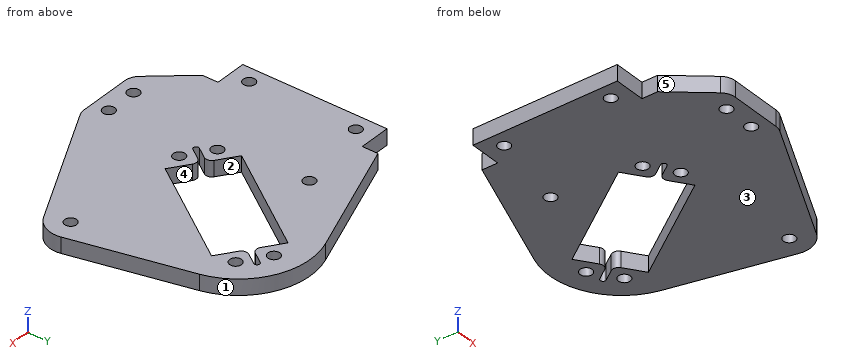
from build123d import *

# Parameters (mm, degrees)
ESQUISSE1_R        = 1.9
BOSS_EXTRU_1_DEPTH = 5


with BuildPart() as part:
    # Esquisse1 → Boss.-Extru.1 (new body)
    with BuildSketch(Plane.XY):
        with BuildLine():
            Line((40.548338426, -21.276277818), (-0.975727052, -42.264773686))
            ThreePointArc((-0.975727052, -42.264773686), (-2.030907408, -42.633295828), (-3.141586831, -42.758217285))
            Line((-3.141586831, -42.758217285), (-19.618188193, -42.758217285))
            ThreePointArc((-19.618188193, -42.758217285), (-21.685859542, -42.310660648), (-23.383370665, -41.048112535))
            Line((-23.383370665, -41.048112535), (-33.519906154, -28.967859949))
            Line((-33.519906154, -28.967859949), (-33.519906154, -23.969415955))
            Line((-33.519906154, -23.969415955), (-43.519906154, -23.969415955))
            Line((-43.519906154, -23.969415955), (-43.519906154, 22.030584045))
            Line((-43.519906154, 22.030584045), (-33.519906154, 22.030584045))
            Line((-33.519906154, 22.030584045), (-33.519906154, 27.030582734))
            Line((-33.519906154, 27.030582734), (5.8804708, 41.371147503))
            ThreePointArc((5.8804708, 41.371147503), (24.71028401, 39.977143129), (36.151646844, 24.957145453))
            Line((36.151646844, 24.957145453), (44.672795688, -12.50542283))
            ThreePointArc((44.672795688, -12.50542283), (44.089997655, -17.586546272), (40.548338426, -21.276277818))
        make_face()
        with Locations((37.968513549, -14.646168575)):
            Circle(ESQUISSE1_R, mode=Mode.SUBTRACT)
        with Locations((26.290921771, 28.768039745)):
            Circle(ESQUISSE1_R, mode=Mode.SUBTRACT)
        with Locations((18.099401328, 34.503804109)):
            Circle(ESQUISSE1_R, mode=Mode.SUBTRACT)
        with Locations((-1.81432361, -11.370410425)):
            Circle(ESQUISSE1_R, mode=Mode.SUBTRACT)
        with Locations((-10.005844053, -5.634646061)):
            Circle(ESQUISSE1_R, mode=Mode.SUBTRACT)
        with Locations((-13.38853652, 21.030583318)):
            Circle(ESQUISSE1_R, mode=Mode.SUBTRACT)
        with Locations((-6.818359545, -37.758216658)):
            Circle(ESQUISSE1_R, mode=Mode.SUBTRACT)
        with Locations((-16.818359545, -37.758216658)):
            Circle(ESQUISSE1_R, mode=Mode.SUBTRACT)
        with Locations((-38.519906154, -17.969415955)):
            Circle(ESQUISSE1_R, mode=Mode.SUBTRACT)
        with Locations((-38.519906154, 16.030584045)):
            Circle(ESQUISSE1_R, mode=Mode.SUBTRACT)
        with BuildLine():
            Line((21.617307412, 29.328732493), (24.05500749, 32.810128977))
            ThreePointArc((24.05500749, 32.810128977), (23.766600359, 33.932469516), (22.625252159, 33.732091761))
            Line((22.625252159, 33.732091761), (20.187552449, 30.250695803))
            ThreePointArc((20.187552449, 30.250695803), (18.892160946, 29.381199086), (17.366350313, 29.706722658))
            Line((17.366350313, 29.706722658), (11.508582376, 33.808377058))
            Line((11.508582376, 33.808377058), (-11.606548602, 0.796549047))
            Line((-11.606548602, 0.796549047), (-5.749613357, -3.304522496))
            ThreePointArc((-5.749613357, -3.304522496), (-4.927150936, -4.595530225), (-5.258462389, -6.089979325))
            Line((-5.258462389, -6.089979325), (-7.696162511, -9.571375872))
            ThreePointArc((-7.696162511, -9.571375872), (-7.487422906, -10.755197269), (-6.303601509, -10.546457664))
            Line((-6.303601509, -10.546457664), (-3.865901833, -7.065061754))
            ThreePointArc((-3.865901833, -7.065061754), (-2.574894061, -6.242599111), (-1.080444801, -6.573910562))
            Line((-1.080444801, -6.573910562), (4.776491193, -10.67498149))
            Line((4.776491193, -10.67498149), (27.891620971, 22.336844808))
            Line((27.891620971, 22.336844808), (22.031293977, 26.440291454))
            ThreePointArc((22.031293977, 26.440291454), (21.198678089, 27.79484445), (21.617307412, 29.328732493))
        make_face(mode=Mode.SUBTRACT)
    extrude(amount=BOSS_EXTRU_1_DEPTH)


solid = part.part
Can you work these out from the model? Positions are in its coordinate system, mm. Face numbers are marked on the shaded views. A direction names the side the tool comes from. Coordinates: 2 decimals unless noted, no trailing zeros. Order: outer loops, then holes, each group sorted by start corner. A loop starts at its lowest first (then second) coordinate and runs counter-clockwise, first axis right, second up. Notation, with made-up numbers: (-35.75, 30.25) -> (1.25, 30.25) arc R36 cw to (1.25, 65.25) -> close; hole circle Ø6 at (15, 56.25). An arc over 180 degrees is marked (long way). Use one line per item in the form item = value.
Q1. Imagine slicing it at A-A, the plane y = 5. List the corners of the cut face in (x, z) for me, then the cut area to 3 significant figures.
From the geometry:
outline = (-43.52, 0) -> (-8.66, 0) -> (-8.66, 5) -> (-43.52, 5) -> close; (15.75, 0) -> (40.69, 0) -> (40.69, 5) -> (15.75, 5) -> close
area = 299 mm²
Q2. We'd pull the mould along X, two halves only. Please class the marked faces 3, 4 and 5: released by +X, released by -X, zero draft, split by the parting line, or undercut.
From the geometry:
face_3 = zero draft
face_4 = undercut
face_5 = released by -X
Q3. Imagine slicing it at C-C, the plane x = -29.5. List the corners of the cut face in (y, z) for me.
From the geometry:
outline = (-33.76, 0) -> (28.49, 0) -> (28.49, 5) -> (-33.76, 5) -> close
Q4. I need wall thicknesses on L1, parallel to Y at x = -38.5, z = 1.9; L2, parallel to Y at x = -37, z = 3.3; L3, parallel to X at y = 21, z = 2.95. Which ranges of each line are inside material? Lowest first, please.
From the geometry:
L1 = -23.97 to -19.87, -16.07 to 14.13, 17.93 to 22.03
L2 = -23.97 to -19.11, -16.83 to 14.89, 17.17 to 22.03
L3 = -43.52 to -15.29, -11.49 to 2.54, 26.96 to 37.05
Q5. Imagine slicing it at D-D, the plane z = 1.7. Give the number of separate pieces and of enclosed holes in the cut face, then the cut area to 3 significant figures.
From the geometry:
separate_pieces = 1
enclosed_holes = 11
area = 4,810 mm²
Q6. Will these pins go through, and if not, where does the flat tip stop? P1, Ø3, axis at x = -38.52, y = 16.03, coming from the +Z side; P2, Ø2.5, axis at x = -37, z = 2, coming from the -Y side; P3, Ø1.5, axis at x = -19.5, z = 4, coming from the +Y side; P4, Ø1.5, axis at x = -40, z = 2, coming from the +Y side.
From the geometry:
P1 = through
P2 = -23.97
P3 = 32.41
P4 = 22.03
Q7. Imagine slicing it at B-B, the plane x = 15. List the corners of the cut face in (y, z) for me, then the cut area to 3 significant figures.
From the geometry:
outline = (-34.19, 0) -> (3.93, 0) -> (3.93, 5) -> (-34.19, 5) -> close; (31.36, 0) -> (42.72, 0) -> (42.72, 5) -> (31.36, 5) -> close
area = 247 mm²
Q8. Which directions (+Z, -Z, +X, -X, +Y, -Y) give clear straight access to the entire face, cutting with the end or side of a thin tool? Please do the marked faces 1 and 2.
From the geometry:
face_1 = +Z, -Z, +Y
face_2 = +Z, -Z
